Check sheet for the modelled part. Datum: model origin and axes. Units: mm. A direction names the side the tool comes from. Round coordinates to 2 decimals unless told otherwise and drop trailing zeros. Write each loop counter-clockwise with the first axis right and the second up, starting at its lowest first coordinate (ties: lowest second). Pieces come first, ordered by that corner, then holes. Notation, with made-up numbers: M 61,-7 L 67,-7 A29 cw 67,13 Z; hole C 77,28 d6. An arc over 180 degrees is marked long. Answer in a Markdown table with one row per item.
```python
from build123d import *

# Parameters (mm, degrees)
F0_W     = 1.5
F0_H     = 5
F0_W_2   = 3
F0_H_2   = 2
F0_H_3   = 3
F1_DEPTH = 3


# Not quite as in the source:
# - a feature names something its author has since deleted; it is built from what else it names


with BuildPart() as f1:
    # F0 (on Front) → F1 (new body)
    with BuildSketch(Plane.XZ):
        with Locations((0.75, 2.5)):
            Rectangle(F0_W, F0_H)
        with Locations((-0.75, 2.5)):
            Rectangle(F0_W, F0_H)
        Polygon((1.5, 5), (1.5, 0), (11.5, 0), (14.5, 0), (14.5, 5), (14.5, 10), (11.5, 10), (1.5, 10), align=None)
        with Locations((13, -1)):
            Rectangle(F0_W_2, F0_H_2)
        with Locations((16, -1)):
            Rectangle(F0_W_2, F0_H_2)
        with Locations((16, 2.5)):
            Rectangle(F0_W_2, F0_H)
        with Locations((19, -1)):
            Rectangle(F0_W_2, F0_H_2)
        Polygon((17.5, 5), (17.5, 0), (20.5, 0), (30.5, 0), (30.5, 5), (30.5, 10), (20.5, 10), (17.5, 10), align=None)
        with Locations((13, 11.5)):
            Rectangle(F0_W_2, F0_H_3)
        with Locations((19, 11.5)):
            Rectangle(F0_W_2, F0_H_3)
        with Locations((32, 2.5)):
            Rectangle(F0_W_2, F0_H)
        Polygon((33.5, 5), (33.5, 0), (43.5, 0), (46.5, 0), (46.5, 5), (46.5, 10), (33.5, 10), align=None)
        with Locations((45, -1)):
            Rectangle(F0_W_2, F0_H_2)
        with Locations((48, -1)):
            Rectangle(F0_W_2, F0_H_2)
        with Locations((48, 2.5)):
            Rectangle(F0_W_2, F0_H)
        with Locations((51, -1)):
            Rectangle(F0_W_2, F0_H_2)
        Polygon((49.5, 5), (49.5, 0), (52.5, 0), (62.5, 0), (62.5, 5), (62.5, 10), (49.5, 10), align=None)
        with Locations((64, 2.5)):
            Rectangle(F0_W_2, F0_H)
        Polygon((78.5, 10), (65.5, 10), (65.5, 5), (65.5, 0), (75.5, 0), (78.5, 0), (78.5, 5), align=None)
        with Locations((77, -1)):
            Rectangle(F0_W_2, F0_H_2)
        Polygon((94.5, 10), (81.5, 10), (81.5, 5), (81.5, 0), (84.5, 0), (94.5, 0), (94.5, 5), align=None)
        with Locations((80, 2.5)):
            Rectangle(F0_W_2, F0_H)
        with Locations((80, -1)):
            Rectangle(F0_W_2, F0_H_2)
        with Locations((83, -1)):
            Rectangle(F0_W_2, F0_H_2)
        with Locations((95.25, 2.5)):
            Rectangle(F0_W, F0_H)
        with Locations((96.75, 2.5)):
            Rectangle(F0_W, F0_H)
        Polygon((110.5, 10), (97.5, 10), (97.5, 5), (97.5, 0), (107.5, 0), (110.5, 0), (110.5, 5), align=None)
        Polygon((126.5, 10), (113.5, 10), (113.5, 5), (113.5, 0), (116.5, 0), (126.5, 0), (126.5, 5), align=None)
        with Locations((112, 2.5)):
            Rectangle(F0_W_2, F0_H)
        with Locations((109, -1)):
            Rectangle(F0_W_2, F0_H_2)
        with Locations((112, -1)):
            Rectangle(F0_W_2, F0_H_2)
        with Locations((115, -1)):
            Rectangle(F0_W_2, F0_H_2)
        Polygon((142.5, 10), (129.5, 10), (129.5, 5), (129.5, 0), (139.5, 0), (142.5, 0), (142.5, 5), align=None)
        with Locations((128, 2.5)):
            Rectangle(F0_W_2, F0_H)
        Polygon((158.5, 10), (145.5, 10), (145.5, 5), (145.5, 0), (148.5, 0), (158.5, 0), (158.5, 5), align=None)
        with Locations((144, 2.5)):
            Rectangle(F0_W_2, F0_H)
        with Locations((144, -1)):
            Rectangle(F0_W_2, F0_H_2)
        with Locations((141, -1)):
            Rectangle(F0_W_2, F0_H_2)
        with Locations((147, -1)):
            Rectangle(F0_W_2, F0_H_2)
        with Locations((160, 2.5)):
            Rectangle(F0_W_2, F0_H)
        Polygon((171.5, 10), (161.5, 10), (161.5, 5), (161.5, 0), (171.5, 0), (174.5, 0), (174.5, 5), (174.5, 10), align=None)
        with Locations((173, 11.5)):
            Rectangle(F0_W_2, F0_H_3)
        with Locations((173, -1)):
            Rectangle(F0_W_2, F0_H_2)
        Polygon((180.5, 10), (177.5, 10), (177.5, 5), (177.5, 0), (180.5, 0), (190.5, 0), (190.5, 5), (190.5, 10), align=None)
        with Locations((179, 11.5)):
            Rectangle(F0_W_2, F0_H_3)
        with Locations((176, 2.5)):
            Rectangle(F0_W_2, F0_H)
        with Locations((176, -1)):
            Rectangle(F0_W_2, F0_H_2)
        with Locations((179, -1)):
            Rectangle(F0_W_2, F0_H_2)
        with Locations((191.25, 2.5)):
            Rectangle(F0_W, F0_H)
        with Locations((192.75, 2.5)):
            Rectangle(F0_W, F0_H)
    extrude(amount=F1_DEPTH)


solid = f1.part
```
1. Scan lines: L1, parallel to X at y = -0.6, z = 11.75; L2, parallel to X at y = -2.7, z = -0.5; L3, parallel to Z at x = 129, y = -1.1. Record each from-to range of solid material in increasing order.
Found:
| item | result |
|---|---|
| L1 | x = 11.5 to 14.5, 17.5 to 20.5, 171.5 to 174.5, 177.5 to 180.5 |
| L2 | x = 11.5 to 20.5, 43.5 to 52.5, 75.5 to 84.5, 107.5 to 116.5, 139.5 to 148.5, 171.5 to 180.5 |
| L3 | z = 0 to 5 |
2. Section check B-B, the plane x = 167.5. Record the cut outline in (y, z).
Found:
| item | result |
|---|---|
| outline | M -3,0 L 0,0 L 0,10 L -3,10 Z |
3. Access from +Z, -Z, +X, -X, +Y, -Y to the whole of each face (thin tool, end or side, straight path). Record for faces 1 (the face through (192, -1, 5)), 2 (the face through (95, 0, 4)), 3 (the face through (1.5, -1, 8)), 4 (the face through (64, -1, 5)).
Found:
| item | result |
|---|---|
| face 1 | +Z, +X, +Y, -Y |
| face 2 | +Z, -Z, +X, -X, +Y |
| face 3 | +Z, -X, +Y, -Y |
| face 4 | +Z, +Y, -Y |
4. Section check A-A, the plane z = 7.5. Count the separate pieces of the cut face and the enclosed holes in it, and give its area (3 significant figures).
Found:
| item | result |
|---|---|
| separate pieces | 12 |
| enclosed holes | 0 |
| area | 468 mm2 |
5. Go/stop test with flat-tipped pins: pin 1 (0.9 mm diameter, centred on y = -2, z = 6.5, fed in from -X); pin 2 (0.6 mm diameter, centred on y = -2, z = -0.5, fed in from +X); pin 3 (3 mm diameter, centred on x = 56.5, z = 0.5, fed in from +Y); pin 4 (1.5 mm diameter, centred on y = -2, z = 12, fed in from -X). Record where each tip stops, or that it passes through.
Found:
| item | result |
|---|---|
| pin 1 | stops at x = 1.5 |
| pin 2 | stops at x = 180.5 |
| pin 3 | stops at y = 0 |
| pin 4 | stops at x = 11.5 |
